The model under review builds one solid part; all positions refer to its coordinate system, in mm. Round coordinates to 2 decimals unless told otherwise and drop trailing zeros. Loops run counter-clockwise (first coordinate to the right, second up) from the corner with the lowest first, then second, coordinate; pieces in that order, holes last. Notation, with made-up numbers: (64, 58) - (79, 58) arc R30 ccw to (79, 87) - close; hole circle Ø10 at (-12, 28.25). An arc over 180 degrees is marked (long way). Answer as CSV lines item,"result".
from build123d import *

# Parameters (mm, degrees)
F0_W         = 106
F0_H         = 10
F0_R         = 1.5
F1_DEPTH     = 7
F2_T1_DEPTH  = 17
F2_T3_DEPTH  = 3
F2_T5_DEPTH  = 13
F2_T7_DEPTH  = 109
F2_S11_W     = 2
F2_S11_H     = 2
F2_T12_DEPTH = 2
F2_S17_W     = 2
F2_S17_H     = 2
F2_T18_DEPTH = 2
F3_T1_DEPTH  = 11
F3_T3_DEPTH  = 3
F3_T5_DEPTH  = 107
F3_S9_W      = 2.04
F3_S9_H      = 2.04
F3_T10_DEPTH = 2.04
F3_S15_W     = 2.04
F3_S15_H     = 2.04
F3_T16_DEPTH = 2.04


# Not quite as in the source:
# - a fillet or chamfer that OpenCascade refuses, or shapes differently, is made with other operations: its cross-section is extruded or revolved along the edge and cut away or added


with BuildPart() as f1:
    # F0 (on Front) → F1 (new body)
    with BuildSketch(Plane.XZ):
        with Locations((0, 5)):
            Rectangle(F0_W, F0_H)
        with Locations((-50, 5)):
            Circle(F0_R, mode=Mode.SUBTRACT)
        with Locations((50, 5)):
            Circle(F0_R, mode=Mode.SUBTRACT)
    extrude(amount=F1_DEPTH)

    # F2: fillet of radius 2 on 7 edges, made by hand

    # F2_s2 → F2_t1 (cut)
    with BuildSketch(Plane.XZ.offset(-5)):
        with BuildLine():
            ThreePointArc((51, 0), (52.4142135624, 0.5857864376), (53, 2))
            Line((53, 2), (53, 0))
            Line((53, 0), (51, 0))
        make_face()
        with BuildLine():
            ThreePointArc((-53, 8), (-52.4142135624, 9.4142135624), (-51, 10))
            Line((-51, 10), (-53, 10))
            Line((-53, 10), (-53, 8))
        make_face()
    extrude(amount=F2_T1_DEPTH, mode=Mode.SUBTRACT)

    # F2_s4 → F2_t3 (cut)
    with BuildSketch(Plane.XZ.offset(2)):
        with BuildLine():
            ThreePointArc((53, 8), (52.4142135624, 9.4142135624), (51, 10))
            Line((51, 10), (53, 10))
            Line((53, 10), (53, 8))
        make_face()
    extrude(amount=F2_T3_DEPTH, mode=Mode.SUBTRACT)

    # F2_s6 → F2_t5 (cut)
    with BuildSketch(Plane.XY.offset(-5)):
        with BuildLine():
            ThreePointArc((53, -2), (52.4142135624, -0.5857864376), (51, 0))
            Line((51, 0), (53, 0))
            Line((53, 0), (53, -2))
        make_face()
        with BuildLine():
            ThreePointArc((53, -5), (52.4142135624, -6.4142135624), (51, -7))
            Line((51, -7), (53, -7))
            Line((53, -7), (53, -5))
        make_face()
    extrude(amount=F2_T5_DEPTH, mode=Mode.SUBTRACT)

    # F2_s8 → F2_t7 (cut)
    with BuildSketch(Plane.YZ.offset(-58)):
        with BuildLine():
            ThreePointArc((-2, 10), (-0.5857864376, 9.4142135624), (0, 8))
            Line((0, 8), (0, 10))
            Line((0, 10), (-2, 10))
        make_face()
        with BuildLine():
            ThreePointArc((-5, 10), (-6.4142135624, 9.4142135624), (-7, 8))
            Line((-7, 8), (-7, 10))
            Line((-7, 10), (-5, 10))
        make_face()
    extrude(amount=F2_T7_DEPTH, mode=Mode.SUBTRACT)


with BuildPart() as f2_tool10:
    # F2_s11 → F2_t12 (new body)
    with BuildSketch(Plane.YZ.offset(51)):
        with Locations((-1, 9)):
            Rectangle(F2_S11_W, F2_S11_H)
    extrude(amount=F2_T12_DEPTH)

    # F2_s13 → F2_t14 (revolve, cut)
    with BuildSketch(Plane(origin=(51, -2, 8), x_dir=(0, -0.7071067812, -0.7071067812), z_dir=(0, -0.7071067812, 0.7071067812))):
        with BuildLine():
            ThreePointArc((0, -2), (2, 0), (0, 2))
            Line((0, 2), (0, -2))
        make_face()
    revolve(axis=Axis((51, -2, 8), (1, 0, 0)), mode=Mode.SUBTRACT)


with BuildPart() as f1_1:
    add(f1.part)

    # F2_t9: cut F2_tool10
    add(f2_tool10.part, mode=Mode.SUBTRACT)


with BuildPart() as f2_tool16:
    # F2_s17 → F2_t18 (new body)
    with BuildSketch(Plane.YZ.offset(51)):
        with Locations((-6, 9)):
            Rectangle(F2_S17_W, F2_S17_H)
    extrude(amount=F2_T18_DEPTH)

    # F2_s19 → F2_t20 (revolve, cut)
    with BuildSketch(Plane(origin=(51, -5, 8), x_dir=(0, 0.7071067812, -0.7071067812), z_dir=(0, -0.7071067812, -0.7071067812))):
        with BuildLine():
            ThreePointArc((0, -2), (2, 0), (0, 2))
            Line((0, 2), (0, -2))
        make_face()
    revolve(axis=Axis((51, -5, 8), (1, 0, 0)), mode=Mode.SUBTRACT)


with BuildPart() as f1_2:
    add(f1_1.part)

    # F2_t15: cut F2_tool16
    add(f2_tool16.part, mode=Mode.SUBTRACT)

    # F3: fillet of radius 2 on 7 edges, made by hand

    # F3_s2 → F3_t1 (cut)
    with BuildSketch(Plane.XY.offset(2)):
        with BuildLine():
            ThreePointArc((-53, -2), (-52.4142135624, -0.5857864376), (-51, 0))
            Line((-51, 0), (-53, 0))
            Line((-53, 0), (-53, -2))
        make_face()
        with BuildLine():
            ThreePointArc((-53, -5), (-52.4142135624, -6.4142135624), (-51, -7))
            Line((-51, -7), (-53, -7))
            Line((-53, -7), (-53, -5))
        make_face()
    extrude(amount=F3_T1_DEPTH, mode=Mode.SUBTRACT)

    # F3_s4 → F3_t3 (cut)
    with BuildSketch(Plane.XZ.offset(2)):
        with BuildLine():
            ThreePointArc((-53, 2), (-52.4142135624, 0.5857864376), (-51, 0))
            Line((-51, 0), (-53, 0))
            Line((-53, 0), (-53, 2))
        make_face()
    extrude(amount=F3_T3_DEPTH, mode=Mode.SUBTRACT)

    # F3_s6 → F3_t5 (cut)
    with BuildSketch(Plane.YZ.offset(-51)):
        with BuildLine():
            ThreePointArc((0, 2), (-0.5857864376, 0.5857864376), (-2, 0))
            Line((-2, 0), (0, 0))
            Line((0, 0), (0, 2))
        make_face()
        with BuildLine():
            ThreePointArc((-5, 0), (-6.4142135624, 0.5857864376), (-7, 2))
            Line((-7, 2), (-7, 0))
            Line((-7, 0), (-5, 0))
        make_face()
    extrude(amount=F3_T5_DEPTH, mode=Mode.SUBTRACT)


with BuildPart() as f3_tool8:
    # F3_s9 → F3_t10 (new body)
    with BuildSketch(Plane.YZ.offset(-51)):
        with Locations((-0.98, 0.98)):
            Rectangle(F3_S9_W, F3_S9_H)
    extrude(amount=-F3_T10_DEPTH)

    # F3_s11 → F3_t12 (revolve, cut)
    with BuildSketch(Plane(origin=(-51, -2, 2), x_dir=(0, -0.7071067812, 0.7071067812), z_dir=(0, -0.7071067812, -0.7071067812))):
        with BuildLine():
            ThreePointArc((0, -2), (2, 0), (0, 2))
            Line((0, 2), (0, -2))
        make_face()
    revolve(axis=Axis((-51, -2, 2), (-1, 0, 0)), mode=Mode.SUBTRACT)


with BuildPart() as f1_3:
    add(f1_2.part)

    # F3_t7: cut F3_tool8
    add(f3_tool8.part, mode=Mode.SUBTRACT)


with BuildPart() as f3_tool14:
    # F3_s15 → F3_t16 (new body)
    with BuildSketch(Plane.YZ.offset(-51)):
        with Locations((-6.02, 0.98)):
            Rectangle(F3_S15_W, F3_S15_H)
    extrude(amount=-F3_T16_DEPTH)

    # F3_s17 → F3_t18 (revolve, cut)
    with BuildSketch(Plane(origin=(-51, -5, 2), x_dir=(0, 0.7071067812, 0.7071067812), z_dir=(0, -0.7071067812, 0.7071067812))):
        with BuildLine():
            ThreePointArc((0, -2), (2, 0), (0, 2))
            Line((0, 2), (0, -2))
        make_face()
    revolve(axis=Axis((-51, -5, 2), (-1, 0, 0)), mode=Mode.SUBTRACT)


with BuildPart() as f1_4:
    add(f1_3.part)

    # F3_t13: cut F3_tool14
    add(f3_tool14.part, mode=Mode.SUBTRACT)


solid = f1_4.part
1. Take a section at A-A (x = -50). State the section outline as (y, z) points, plus the area to 3 significant figures.
Numbers:
outline,"(-7, 2) arc R2 ccw to (-5, 0) - (-2, 0) arc R2 ccw to (0, 2) - (0, 3.5) - (-7, 3.5) - close; (-7, 6.5) - (0, 6.5) - (0, 8) arc R2 ccw to (-2, 10) - (-5, 10) arc R2 ccw to (-7, 8) - close"
area,"45.6 mm²"
2. Take a section at B-B (y = -4). State the section outline as (x, z) points, plus the area to 3 significant figures.
Numbers:
outline,"(-53, 2) arc R2 ccw to (-51, 0) - (51, 0) arc R2 ccw to (53, 2) - (53, 8) arc R2 ccw to (51, 10) - (-51, 10) arc R2 ccw to (-53, 8) - close; hole circle Ø3 at (-50, 5); hole circle Ø3 at (50, 5)"
area,"1,040 mm²"
3. Draft analysis for pull direction Z (two halves, no side actions). For faces 1 (the face through (48.5, -3.45, 5.07)), 2 (the face through (-1, -3, 10)), 3 (the face through (-53, -3, 5)), state which applies: +Z half, -Z half, draft (parallel to the pull), parting line (faces both ways), or undercut.
Numbers:
face 1,"undercut"
face 2,"+Z half"
face 3,"draft"
4. Take a section at D-D (x = 17). State the section outline as (y, z) points.
Numbers:
outline,"(-7, 2) arc R2 ccw to (-5, 0) - (-2, 0) arc R2 ccw to (0, 2) - (0, 8) arc R2 ccw to (-2, 10) - (-5, 10) arc R2 ccw to (-7, 8) - close"
5. Wall thickness on probe 1 along Z at (x, y) = (-50, -4.5); probe 2 along X at (y, z) = (-0.5, 6); probe 3 along Z at (x, y) = (-26.5, -1.75): over which ranges is each line inside the solid? List them lowest first.
Numbers:
probe 1,"z = 0 to 3.5, 6.5 to 10"
probe 2,"x = -52.32 to -51.12, -48.88 to 48.88, 51.12 to 52.32"
probe 3,"z = 0.02 to 9.98"
6. Take a section at C-C (z = 5). State the section outline as (x, y) points, plus the area to 3 significant figures.
Numbers:
outline,"(-53, -5) arc R2 ccw to (-51.5, -6.94) - (-51.5, -0.06) arc R2 ccw to (-53, -2) - close; (-48.5, -7) - (48.5, -7) - (48.5, 0) - (-48.5, 0) - close; (51.5, -6.94) arc R2 ccw to (53, -5) - (53, -2) arc R2 ccw to (51.5, -0.06) - close"
area,"697 mm²"
